For this review, take the finished solid that the model builds, in its own axes (mm). A direction names the side the tool comes from. Round coordinates to 2 decimals unless told otherwise and drop trailing zeros. Loops run counter-clockwise (first coordinate to the right, second up) from the corner with the lowest first, then second, coordinate; pieces in that order, holes last.
1. Draft analysis for pull direction X (two halves, no side actions). For faces 6 (the flat face through (8, 2.7, 1)), 7 (the flat face through (10.725, -3, 0)), 8 (the flat face through (-4, 0, -3)), state which applies: released by +X, released by -X, zero draft, split by the parting line, or undercut.
2. To check wall thickness, follow line 1 along Z through (x, y) = (14, -5.5) (3 decimals); line 2 along X through (y, z) = (-5.5, -4.5) (3 decimals); line 3 along Z through (x, y) = (-3.5, -4.25) (3 decimals). State the ranges of each line that lie inside material, in increasing order.
3. Consider section A-A on x = 3.5. State the section outline as (y, z) points (3 decimals), then the cut area to 3 significant figures.
4. Tool access review of faces 1 (the flat face through (-12.5, -3.25, -0.7)), 2 (the flat face through (-2.725, -2, 0.5)), 3 (the cylindrical face through (-11.67, -2.92, -2.93)), 4 (the flat face through (13, -5.2, 0)), 5 (the cylindrical face through (17.859, 0.74, -3.634)): name each direction out of +Z, -Z, +X, -X, +Y, -Y from which nothing blocks a thin tool from reaching the whole face with its end or side.
5. Consider section B-B on y = -1.25. State how many separate pieces and enclosed holes the cut face has, then the cut area to 3 significant figures.
6. Consider section D-D on x = -4. State the section outline as (y, z) points (3 decimals), then the cut area to 3 significant figures.
7. Consider section C-C on x = -11. State the section outline as (y, z) points (3 decimals).
8. Clearance check with flat-ended pins moving along their axes: pin 1 Ø2 at (x, z) = (-15, -4) entering from +Y; pin 2 Ø0.6 at (y, z) = (-5.5, 1.5) entering from +X (3 decimals); pin 3 Ø2.5 at (x, z) = (-4.195, -2.975) entering from -Y. State where each tip first meets the part, or that it passes through.
from build123d import *

# Parameters (mm, degrees)
SKETCH1_W           = 39.71
SKETCH1_H           = 16.25
SKETCH1_R           = 1.85
BOSS_EXTRUDE1_DEPTH = 1.5
SKETCH2_W           = 6.9
SKETCH2_H           = 12.5
BOSS_EXTRUDE2_DEPTH = 5.9
CUT_EXTRUDE1_DEPTH  = 5
SKETCH3_3_W         = 0.7
SKETCH3_3_H         = 1
SKETCH3_3_W_2       = 1
SKETCH3_3_H_2       = 0.7
CUT_EXTRUDE2_DEPTH  = 3.6
BOSS_EXTRUDE3_DEPTH = 5.75
SKETCH6_R           = 1.075
CUT_EXTRUDE3_DEPTH  = 5.75
SKETCH4_3_W         = 0.83
SKETCH4_3_H         = 2.45
BOSS_EXTRUDE4_DEPTH = 3.25
CUT_EXTRUDE4_DEPTH  = 11
BOSS_EXTRUDE5_DEPTH = 2.07
SKETCH11_R          = 0.5
BOSS_EXTRUDE6_DEPTH = 1.2
SKETCH11_3_R        = 0.5
BOSS_EXTRUDE7_DEPTH = 0.2


with BuildPart() as part:
    # Sketch1 → Boss-Extrude1 (new body)
    with BuildSketch(Plane(origin=(0, 0, 0), x_dir=(1, 0, 0), z_dir=(0, 1, 0))):
        Rectangle(SKETCH1_W, SKETCH1_H)
        with Locations((17.005, 5.275)):
            Circle(SKETCH1_R, mode=Mode.SUBTRACT)
        with Locations((17.005, -5.275)):
            Circle(SKETCH1_R, mode=Mode.SUBTRACT)
        with Locations((2.105, 5.275)):
            Circle(SKETCH1_R, mode=Mode.SUBTRACT)
        with Locations((-16.895, 5.275)):
            Circle(SKETCH1_R, mode=Mode.SUBTRACT)
    extrude(amount=BOSS_EXTRUDE1_DEPTH)

    # Sketch2 → Boss-Extrude2 (add)
    with BuildSketch(Plane.XZ):
        with Locations((12.275, 0)):
            Rectangle(SKETCH2_W, SKETCH2_H)
    extrude(amount=BOSS_EXTRUDE2_DEPTH)

    # Sketch3 → Cut-Extrude1 (cut)
    with BuildSketch(Plane(origin=(15.725, 0, 0), x_dir=(0, 0, -1), z_dir=(1, 0, 0))):
        Polygon((5.55, -0.7), (3.939297937, -0.7), (-3.939297937, -0.7), (-5.55, -0.7), (-5.55, -5.2), (5.55, -5.2), align=None)
    extrude(amount=-CUT_EXTRUDE1_DEPTH, mode=Mode.SUBTRACT)

    # Sketch3<3> → Cut-Extrude2 (cut)
    with BuildSketch(Plane(origin=(15.725, 0, 0), x_dir=(0, 0, -1), z_dir=(1, 0, 0))):
        with Locations((-5.9, -4.7)):
            Rectangle(SKETCH3_3_W, SKETCH3_3_H)
        with Locations((-3.225, -5.55)):
            Rectangle(SKETCH3_3_W_2, SKETCH3_3_H_2)
        with Locations((3.225, -5.55)):
            Rectangle(SKETCH3_3_W_2, SKETCH3_3_H_2)
        with Locations((5.9, -4.7)):
            Rectangle(SKETCH3_3_W, SKETCH3_3_H)
    extrude(amount=-CUT_EXTRUDE2_DEPTH, mode=Mode.SUBTRACT)

    # Sketch4 → Boss-Extrude3 (add)
    with BuildSketch(Plane.XZ):
        Polygon((-12.895, -1.575), (-13.825, -1.575), (-13.825, -8.125), (-0.965, -8.125), (-0.965, -1.575), (-1.895, -1.575), (-2.725, -1.575), (-6.98, -1.575), (-7.81, -1.575), (-12.065, -1.575), align=None)
    extrude(amount=BOSS_EXTRUDE3_DEPTH)

    # Sketch6 → Cut-Extrude3 (cut)
    with BuildSketch(Plane.XZ.offset(5.75)):
        with Locations((-10.595, -2.975)):
            Circle(SKETCH6_R)
        with Locations((-4.195, -2.975)):
            Circle(SKETCH6_R)
    extrude(amount=-CUT_EXTRUDE3_DEPTH, mode=Mode.SUBTRACT)

    # Sketch4<3> → Boss-Extrude4 (add)
    with BuildSketch(Plane.XZ):
        with Locations((-12.48, -0.35)):
            Rectangle(SKETCH4_3_W, SKETCH4_3_H)
        with Locations((-7.395, -0.35)):
            Rectangle(SKETCH4_3_W, SKETCH4_3_H)
        with Locations((-2.31, -0.35)):
            Rectangle(SKETCH4_3_W, SKETCH4_3_H)
    extrude(amount=BOSS_EXTRUDE4_DEPTH)

    # Sketch9 → Cut-Extrude4 (cut)
    with BuildSketch(Plane.ZY.offset(12.895)):
        with BuildLine():
            Line((-1.575, 0), (0.325, 0))
            Line((0.325, 0), (0.325, -2.6))
            ThreePointArc((0.325, -2.6), (0.295710678, -2.670710678), (0.225, -2.7))
            Line((0.225, -2.7), (-1.575, -2.7))
            Line((-1.575, -2.7), (-1.575, 0))
        make_face()
        with BuildLine():
            Line((0.875, -2.6), (0.875, -3.25))
            Line((0.875, -3.25), (0.225, -3.25))
            ThreePointArc((0.225, -3.25), (0.684619408, -3.059619408), (0.875, -2.6))
        make_face()
    extrude(amount=-CUT_EXTRUDE4_DEPTH, mode=Mode.SUBTRACT)

    # Sketch10 → Boss-Extrude5 (add, symmetric)
    with BuildSketch(Plane(origin=(0, -2.875, 0), x_dir=(-1, 0, 0), z_dir=(0, -1, 0))):
        with BuildLine():
            Line((1.965, 8.125), (1.965, 8.225))
            Line((1.965, 8.225), (13.72492529, 11.596310791))
            ThreePointArc((13.72492529, 11.596310791), (13.820005869, 11.634489053), (13.905307898, 11.691246962))
            Line((13.905307898, 11.691246962), (15.087352442, 12.666329881))
            ThreePointArc((15.087352442, 12.666329881), (15.26773505, 12.761266052), (15.471018562, 12.776318482))
            Line((15.471018562, 12.776318482), (17.093348193, 12.561963226))
            Line((17.093348193, 12.561963226), (17.143124243, 12.938689048))
            Line((17.143124243, 12.938689048), (15.520794612, 13.153044304))
            ThreePointArc((15.520794612, 13.153044304), (15.163015631, 13.126552026), (14.84554224, 12.959464366))
            Line((14.84554224, 12.959464366), (13.663497696, 11.984381447))
            ThreePointArc((13.663497696, 11.984381447), (13.643025209, 11.970759549), (13.62020587, 11.961596766))
            Line((13.62020587, 11.961596766), (1.585, 8.511369113))
            Line((1.585, 8.511369113), (1.585, 8.125))
            Line((1.585, 8.125), (1.965, 8.125))
        make_face()
    extrude(amount=BOSS_EXTRUDE5_DEPTH, both=True)

    # Sketch11 → Boss-Extrude6 (add)
    with BuildSketch(Plane(origin=(0, 1.5, 0), x_dir=(1, 0, 0), z_dir=(0, 1, 0))):
        with Locations((-12.48, -0.6)):
            Circle(SKETCH11_R)
        with Locations((-7.395, -0.6)):
            Circle(SKETCH11_R)
        with Locations((-2.31, -0.6)):
            Circle(SKETCH11_R)
        with Locations((8.005, 3.75)):
            Circle(SKETCH11_R)
        with Locations((8.005, 1.25)):
            Circle(SKETCH11_R)
        with Locations((8.005, -1.25)):
            Circle(SKETCH11_R)
        with Locations((8.005, -3.75)):
            Circle(SKETCH11_R)
    extrude(amount=BOSS_EXTRUDE6_DEPTH)

    # Sketch11<3> → Boss-Extrude7 (add)
    with BuildSketch(Plane(origin=(0, 1.5, 0), x_dir=(1, 0, 0), z_dir=(0, 1, 0))):
        with BuildLine():
            Line((-13.48, -1.6), (-13.48, 0.4))
            ThreePointArc((-13.48, 0.4), (-12.48, 1.4), (-11.48, 0.4))
            Line((-11.48, 0.4), (-11.48, -1.6))
            ThreePointArc((-11.48, -1.6), (-12.48, -2.6), (-13.48, -1.6))
        make_face()
        with Locations((-12.48, -0.6)):
            Circle(SKETCH11_3_R, mode=Mode.SUBTRACT)
        with BuildLine():
            Line((-8.395, -1.6), (-8.395, 0.4))
            ThreePointArc((-8.395, 0.4), (-7.395, 1.4), (-6.395, 0.4))
            Line((-6.395, 0.4), (-6.395, -1.6))
            ThreePointArc((-6.395, -1.6), (-7.395, -2.6), (-8.395, -1.6))
        make_face()
        with Locations((-7.395, -0.6)):
            Circle(SKETCH11_3_R, mode=Mode.SUBTRACT)
        with BuildLine():
            Line((-3.31, -1.6), (-3.31, 0.4))
            ThreePointArc((-3.31, 0.4), (-2.31, 1.4), (-1.31, 0.4))
            Line((-1.31, 0.4), (-1.31, -1.6))
            ThreePointArc((-1.31, -1.6), (-2.31, -2.6), (-3.31, -1.6))
        make_face()
        with Locations((-2.31, -0.6)):
            Circle(SKETCH11_3_R, mode=Mode.SUBTRACT)
        with BuildLine():
            Line((7.155, 4.65), (8.855, 4.65))
            ThreePointArc((8.855, 4.65), (9.755, 3.75), (8.855, 2.85))
            Line((8.855, 2.85), (7.155, 2.85))
            ThreePointArc((7.155, 2.85), (6.255, 3.75), (7.155, 4.65))
        make_face()
        with Locations((8.005, 3.75)):
            Circle(SKETCH11_3_R, mode=Mode.SUBTRACT)
        with BuildLine():
            Line((7.155, 2.15), (8.855, 2.15))
            ThreePointArc((8.855, 2.15), (9.755, 1.25), (8.855, 0.35))
            Line((8.855, 0.35), (7.155, 0.35))
            ThreePointArc((7.155, 0.35), (6.255, 1.25), (7.155, 2.15))
        make_face()
        with Locations((8.005, 1.25)):
            Circle(SKETCH11_3_R, mode=Mode.SUBTRACT)
        with BuildLine():
            Line((7.155, -0.35), (8.855, -0.35))
            ThreePointArc((8.855, -0.35), (9.755, -1.25), (8.855, -2.15))
            Line((8.855, -2.15), (7.155, -2.15))
            ThreePointArc((7.155, -2.15), (6.255, -1.25), (7.155, -0.35))
        make_face()
        with Locations((8.005, -1.25)):
            Circle(SKETCH11_3_R, mode=Mode.SUBTRACT)
        with BuildLine():
            Line((7.155, -2.85), (8.855, -2.85))
            ThreePointArc((8.855, -2.85), (9.755, -3.75), (8.855, -4.65))
            Line((8.855, -4.65), (7.155, -4.65))
            ThreePointArc((7.155, -4.65), (6.255, -3.75), (7.155, -2.85))
        make_face()
        with Locations((8.005, -3.75)):
            Circle(SKETCH11_3_R, mode=Mode.SUBTRACT)
    extrude(amount=BOSS_EXTRUDE7_DEPTH)


solid = part.part
Resolved:
1. face 6: zero draft
1. face 7: released by +X
1. face 8: undercut
2. line 1: z = -6.25 to -3.725, -2.725 to 2.725, 3.725 to 6.25
2. line 2: x = -13.825 to -0.965, 8.825 to 15.725
2. line 3: z = -9.06 to -8.665, -8.125 to -3.795, -2.155 to -1.575
3. outline: (0, -8.125) - (1.5, -8.125) - (1.5, -6.49) - (0, -6.49) - close; (0, -4.06) - (1.5, -4.06) - (1.5, 8.125) - (0, 8.125) - close
3. area: 20.7 mm2
4. face 1: +Z, -X, -Y
4. face 2: +Z, -Y
4. face 3: -Y
4. face 4: +X
4. face 5: +Y
5. separate pieces: 5
5. enclosed holes: 2
5. area: 115 mm2
6. outline: (-5.75, -8.125) - (1.5, -8.125) - (1.5, 8.125) - (0, 8.125) - (0, -1.575) - (-5.75, -1.575) - (-5.75, -1.918) - (0, -1.918) - (0, -4.032) - (-5.75, -4.032) - close; (-4.945, -9.204) - (-0.805, -9.204) - (-0.805, -8.808) - (-4.945, -8.808) - close
6. area: 51.5 mm2
7. outline: (-5.75, -8.125) - (1.5, -8.125) - (1.5, 8.125) - (0, 8.125) - (0, -1.575) - (-5.75, -1.575) - (-5.75, -1.979) - (0, -1.979) - (0, -3.971) - (-5.75, -3.971) - close; (-4.945, -11.21) - (-0.805, -11.21) - (-0.805, -10.815) - (-4.945, -10.815) - close
8. pin 1: stops at y = 1.5
8. pin 2: stops at x = 15.725
8. pin 3: stops at y = -5.75
